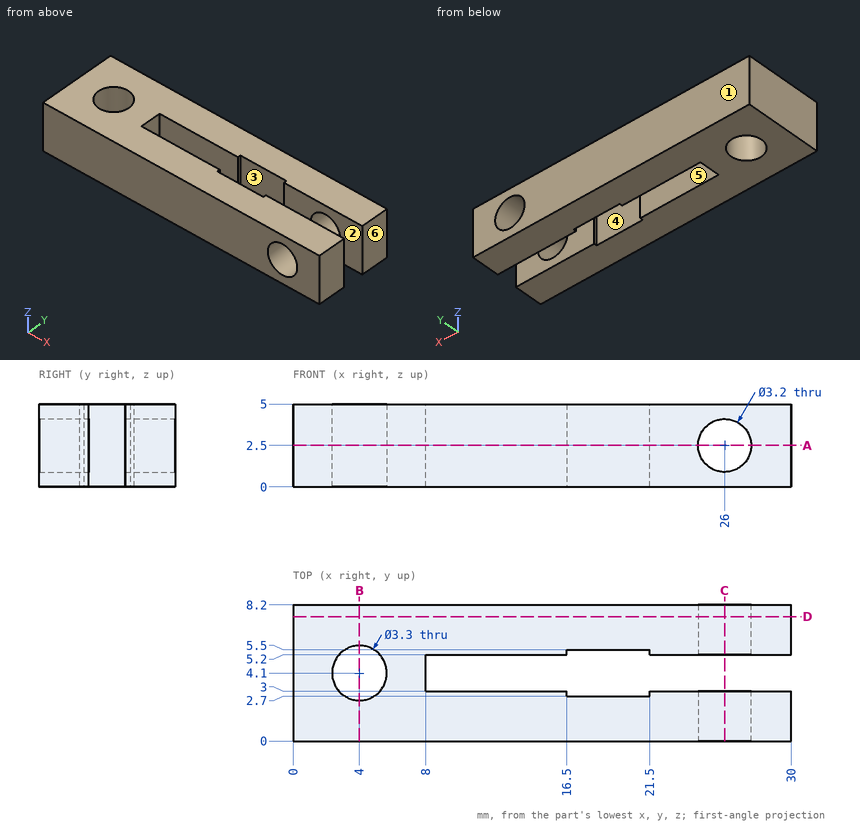
Input: dimensioned drawing with shaded views. Units: mm. Origin: part minimum x, y, z. A direction names the side the tool comes from. Round coordinates to 2 decimals unless told otherwise and drop trailing zeros. Order: outer loops, then holes, each group sorted by start corner. A loop starts at its lowest first (then second) coordinate and runs counter-clockwise, first axis right, second up. Notation, with made-up numbers: (54.25, -24) - (66.25, -24) arc R28 ccw to (66.25, 7) - close; hole circle Ø5 at (24.25, 7). An arc over 180 degrees is marked (long way). Answer as a JSON object with one key per item and string values. Group by question number.
(1) Cut plane B-B (x = 4). Return loops of the section in (y, z).
(2) Cut plane D-D (y = 7.5). Return loops of the section in (x, z).
(3) Cut plane A-A (z = 2.5). Return loops of the section in (x, y).
(4) Reachability of the marked faces 1, 2 and 3 from +Z, -Z, +X, -X, +Y, -Y: full face, straight path, thin tool, end or side. Return the list, or none.
(5) Cut plane C-C (x = 26). Return loops of the section in (y, z), then the cut area to 3 significant figures.
(6) Material intervals for probe 1 along Y at (x, z) = (4, 2.75); probe 2 along Y at (x, z) = (15.5, 0.75); probe 3 along Z at (x, y) = (26, 1.95), sorted ascending. Write a range as from..to.
(7) Draft query along X for the marked faces 4, 5 and 6. Return one class per face: released by +X, released by -X, zero draft, split by the parting line, or undercut.
Here are the results:
{
 "1": {"outline": "(0, 0) - (2.45, 0) - (2.45, 5) - (0, 5) - close; (5.75, 0) - (8.2, 0) - (8.2, 5) - (5.75, 5) - close"},
 "2": {"outline": "(0, 0) - (30, 0) - (30, 5) - (0, 5) - close; hole circle Ø3.2 at (26, 2.5)"},
 "3": {"outline": "(0, 0) - (24.4, 0) - (24.4, 3) - (21.5, 3) - (21.5, 2.7) - (16.5, 2.7) - (16.5, 3) - (8, 3) - (8, 5.2) - (16.5, 5.2) - (16.5, 5.5) - (21.5, 5.5) - (21.5, 5.2) - (24.4, 5.2) - (24.4, 8.2) - (0, 8.2) - close; (27.6, 0) - (30, 0) - (30, 3) - (27.6, 3) - close; (27.6, 5.2) - (30, 5.2) - (30, 8.2) - (27.6, 8.2) - close; hole circle Ø3.3 at (4, 4.1)"},
 "4": {"face 1": "+Z, -Z, +X, -X, +Y", "face 2": "+Z, -Z, +X", "face 3": "+Z, -Z"},
 "5": {"outline": "(0, 0) - (3, 0) - (3, 0.9) - (0, 0.9) - close; (0, 4.1) - (3, 4.1) - (3, 5) - (0, 5) - close; (5.2, 0) - (8.2, 0) - (8.2, 0.9) - (5.2, 0.9) - close; (5.2, 4.1) - (8.2, 4.1) - (8.2, 5) - (5.2, 5) - close", "area": "10.8 mm^2"},
 "6": {"probe 1": "y = 0..2.45, 5.75..8.2", "probe 2": "y = 0..3, 5.2..8.2", "probe 3": "z = 0..0.9, 4.1..5"},
 "7": {"face 4": "undercut", "face 5": "zero draft", "face 6": "released by +X"}
}
